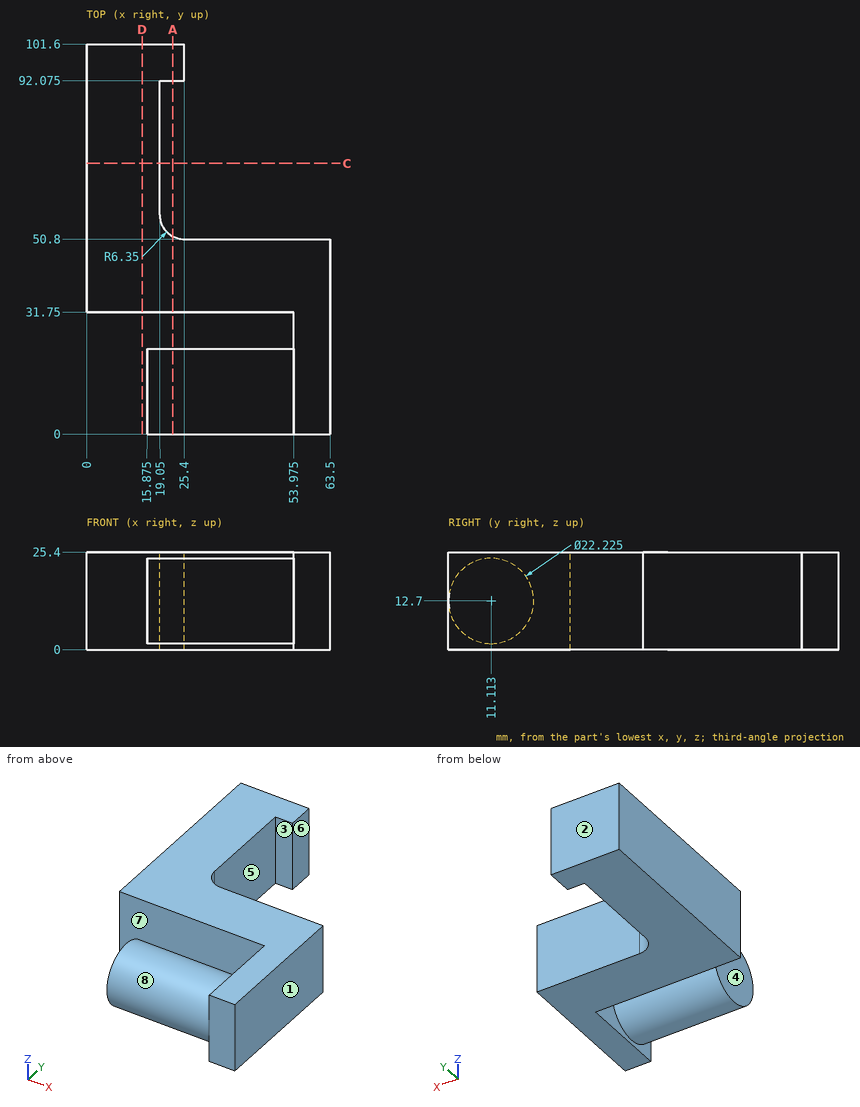
Verification items for this drawing (mm, ordinates from the low corner). A direction names the side the tool comes from. Round coordinates to 2 decimals unless told otherwise and drop trailing zeros. Loops run counter-clockwise (first coordinate to the right, second up) from the corner with the lowest first, then second, coordinate; pieces in that order, holes last. Notation, with made-up numbers: (-13.75, 84) -> (-5.75, 84) arc R24 cw to (-5.75, 103) -> close; hole circle Ø8 at (14.25, -24.75). An arc over 180 degrees is marked (long way). Answer in a Markdown table with one row per item.
Q1. Go/stop test with flat-tipped pins: P1, Ø7.5, axis at y = 72, z = 16, coming from the +X side; P2, Ø4, axis at x = 43, z = 15.5, coming from the +Y side; P3, Ø12.5, axis at y = 8, z = 7, coming from the -X side (1 decimal). Record where each tip stops, or that it passes through.
Data:
| item | result |
|---|---|
| P1 | stops at x = 19.05 |
| P2 | stops at y = 50.8 |
| P3 | stops at x = 15.9 |
Q2. Release check for a two-part mould opening along Y. For the marked faces 1, 2 and 3 record: released by +Y, released by -Y, zero draft, split by the parting line, or undercut.
Data:
| item | result |
|---|---|
| face 1 | zero draft |
| face 2 | released by +Y |
| face 3 | undercut |
Q3. Set-up check for the marked faces 4, 5, 6, 7 and 8: record each of +Z, -Z, +X, -X, +Y, -Y from which the full face is reachable in a straight line by a thin tool's end or side.
Data:
| item | result |
|---|---|
| face 4 | +Z, -Z, -X, -Y |
| face 5 | +Z, -Z, +X |
| face 6 | +Z, -Z, +X, +Y |
| face 7 | +Z, -Z, -X |
| face 8 | -X |
Q4. Sectioned sample at D-D on x = 14.5. Enter the section's corners in (y, z), then the cut area to 3 significant figures.
Data:
| item | result |
|---|---|
| outline | (31.75, 0) -> (101.6, 0) -> (101.6, 25.4) -> (31.75, 25.4) -> close |
| area | 1,770 mm^2 |
Q5. Sectioned sample at C-C on y = 70.5. Enter the section's corners in (x, z), then the cut area to 3 significant figures.
Data:
| item | result |
|---|---|
| outline | (0, 0) -> (19.05, 0) -> (19.05, 25.4) -> (0, 25.4) -> close |
| area | 484 mm^2 |
Q6. Thickness scan on L1, parallel to X at y = 11.5, z = 12.5 (1 decimal); L2, parallel to Y at x = 43, z = 14.5; L3, parallel to X at y = 81, z = 5.25. Record the ranges inside material, lowest first.
Data:
| item | result |
|---|---|
| L1 | x = 15.9 to 63.5 |
| L2 | y = 0.15 to 22.08, 31.75 to 50.8 |
| L3 | x = 0 to 19.05 |
Q7. Sectioned sample at A-A on x = 22.5. Give the number of separate pieces and of enclosed holes in the cut face, then the cut area to 3 significant figures.
Data:
| item | result |
|---|---|
| separate pieces | 3 |
| enclosed holes | 0 |
| area | 1,130 mm^2 |
